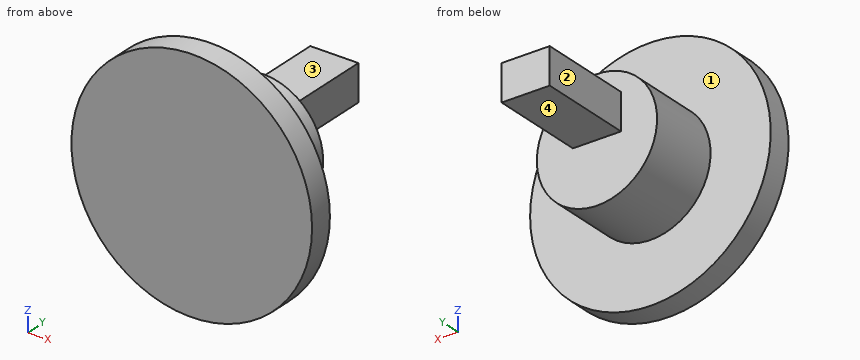
```python
from build123d import *

# Parameters (mm, degrees)
SKETCH1_R           = 5
BOSS_EXTRUDE1_DEPTH = 6
SKETCH3_W           = 4
SKETCH3_H           = 3
BOSS_EXTRUDE2_DEPTH = 8
SKETCH4_R           = 10
BOSS_EXTRUDE3_DEPTH = 2


with BuildPart() as part:
    # Sketch1 → Boss-Extrude1 (new body)
    with BuildSketch(Plane(origin=(0, 0, 0), x_dir=(1, 0, 0), z_dir=(0, 1, 0))):
        Circle(SKETCH1_R)
    extrude(amount=BOSS_EXTRUDE1_DEPTH)

    # Sketch3 → Boss-Extrude2 (add)
    with BuildSketch(Plane(origin=(0, 6, 0), x_dir=(1, 0, 0), z_dir=(0, 1, 0))):
        with Locations((0, -1.5)):
            Rectangle(SKETCH3_W, SKETCH3_H)
    extrude(amount=BOSS_EXTRUDE2_DEPTH)

    # Sketch4 → Boss-Extrude3 (add)
    with BuildSketch(Plane.XZ):
        Circle(SKETCH4_R)
    extrude(amount=BOSS_EXTRUDE3_DEPTH)


solid = part.part
```
Here's how the part is built. I have some questions about the finished solid (model axes, mm). Face numbers are marked on the shaded views. A direction names the side the tool comes from. Round coordinates to 2 decimals unless told otherwise and drop trailing zeros. Order: outer loops, then holes, each group sorted by start corner. A loop starts at its lowest first (then second) coordinate and runs counter-clockwise, first axis right, second up. Notation, with made-up numbers: (75.5, 14) -> (128.5, 14) arc R20 ccw to (128.5, 41) -> close; hole circle Ø8 at (-25.75, 85.25). An arc over 180 degrees is marked (long way). Use a Markdown table: item, result. Add a question column.
(1) Suppose I cut it at C-C, the plane y = 9. Please give me the cut outline in (x, z), and give its area (3 significant figures).
(2) For the marked faces 1, 2, 3 and 4, which set-ups out of +Z, -Z, +X, -X, +Y, -Y let a thin tool reach every point of the face, with its end or its side?
(3) Suppose I cut it at D-D, the plane x = -2.75. Please give me the cut outline in (y, z), and give its area (3 significant figures).
(4) Suppose I cut it at A-A, the plane z = 2. Please give me the cut outline in (x, y), and give its area (3 significant figures).
(5) For pin 1 Ø5 at (x, z) = (-3, 3) entering from +Y; pin 2 Ø2 at (x, y) = (0, 11.5) entering from -Z; pin 3 Ø1 at (y, z) = (4.5, 0) entering from -X; pin 4 Ø2 at (x, y) = (0, 8.5) entering from +Z, each with a flat end and sliding along its axis, tell me the tip position at first contact or that it passes through.
(6) Suppose I cut it at B-B, the plane x = 0. Please give me the cut outline in (y, z).
(7) I need wall thicknesses on line 1 along Y through (x, z) = (-8.5, -3); line 2 along Y through (x, z) = (-2.5, -2.5); line 3 along Z through (x, y) = (-0.75, 1.5). Which ranges of each line are inside material? Lowest first, please.
Verdict:
| question | item | result |
|---|---|---|
| 1 | outline | (-2, 0) -> (2, 0) -> (2, 3) -> (-2, 3) -> close |
| 1 | area | 12.0 mm2 |
| 2 | face 1 | +Y |
| 2 | face 2 | +Z, -Z, -X, +Y |
| 2 | face 3 | +Z, +X, -X, +Y |
| 2 | face 4 | -Z, +X, -X, +Y |
| 3 | outline | (-2, -9.61) -> (0, -9.61) -> (0, -4.18) -> (6, -4.18) -> (6, 4.18) -> (0, 4.18) -> (0, 9.61) -> (-2, 9.61) -> close |
| 3 | area | 88.6 mm2 |
| 4 | outline | (-9.8, -2) -> (9.8, -2) -> (9.8, 0) -> (4.58, 0) -> (4.58, 6) -> (2, 6) -> (2, 14) -> (-2, 14) -> (-2, 6) -> (-4.58, 6) -> (-4.58, 0) -> (-9.8, 0) -> close |
| 4 | area | 126 mm2 |
| 5 | pin 1 | y = 14 |
| 5 | pin 2 | z = 0 |
| 5 | pin 3 | x = -5 |
| 5 | pin 4 | z = 3 |
| 6 | outline | (-2, -10) -> (0, -10) -> (0, -5) -> (6, -5) -> (6, 0) -> (14, 0) -> (14, 3) -> (6, 3) -> (6, 5) -> (0, 5) -> (0, 10) -> (-2, 10) -> close |
| 7 | line 1 | -2 to 0 |
| 7 | line 2 | -2 to 6 |
| 7 | line 3 | -4.94 to 4.94 |
